Source: three-view drawing plus pictorial views. Frame: mm from the lowest corner of the part. A direction names the side the tool comes from. Round coordinates to 2 decimals unless told otherwise and drop trailing zeros. Loops run counter-clockwise (first coordinate to the right, second up) from the corner with the lowest first, then second, coordinate; pieces in that order, holes last. Notation, with made-up numbers: (29, 30) -> (66, 30) arc R27 ccw to (66, 49) -> close; hole circle Ø3 at (31.5, 58). An arc over 180 degrees is marked (long way). One line per question, with ' | ' between items. Start each with the question number.
Q1. Cut plane B-B on x = 17. Return loops of the section in (y, z).
Q2. Material intervals for L1, parallel to X at y = 2.25, z = 11.75; L2, parallel to Z at x = 21.75, y = 7.5; L3, parallel to Z at x = 9.5, y = 2.5, sorted ascending.
Q3. Access query for the marked faces 1, 2 and 3. Directions: +Z, -Z, +X, -X, +Y, -Y. A direction counts if a zero-diameter tool reaches every point of the face in a straight line with its end or side. Return the directions, or none.
Q4. Cut plane C-C on z = 4.75. Return loops of the section in (x, y).
Q5. Mould query, pull axis X, two halves, no side actions, for the marked faces 4, 5, 6 and 7. Classes: pulls with the +X half, pulls with the -X half, needs draft (parallel to the pull), parting line crosses it, or undercut.
Q6. Contact query for flat-ended pins moving along their axis: P1, Ø3.5, axis at y = 9.5, z = 7.5, coming from the -X side; P2, Ø1.5, axis at x = 2.5, z = 15.5, coming from the +Y side; P3, Ø1.5, axis at x = 11.5, z = 12, coming from the +Y side; P4, Ø6, axis at x = 15.5, y = 4.5, coming from the -Z side. Output: stop coordinate, or through.
Q7. Cut plane A-A on y = 5. Return loops of the section in (x, z), and give its area (3 significant figures).
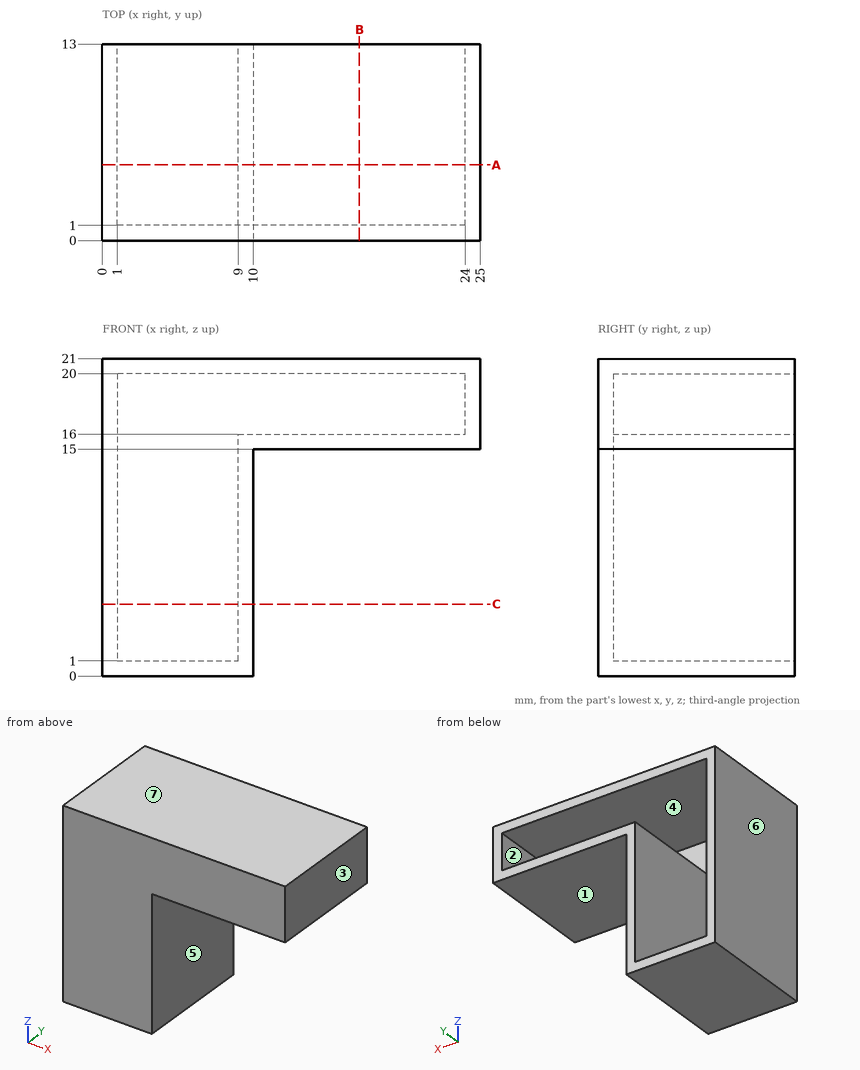
Results:
1) outline: (0, 15) -> (13, 15) -> (13, 16) -> (1, 16) -> (1, 20) -> (13, 20) -> (13, 21) -> (0, 21) -> close
2) L1: 0 to 1, 9 to 10 | L2: 15 to 16, 20 to 21 | L3: 0 to 16, 20 to 21
3) face 1: -Z, +X, +Y, -Y | face 2: +Y | face 3: +Z, -Z, +X, +Y, -Y
4) outline: (0, 0) -> (10, 0) -> (10, 13) -> (9, 13) -> (9, 1) -> (1, 1) -> (1, 13) -> (0, 13) -> close
5) face 4: undercut | face 5: pulls with the +X half | face 6: pulls with the -X half | face 7: needs draft
6) P1: x = 0 | P2: y = 1 | P3: through | P4: z = 15
7) outline: (0, 0) -> (10, 0) -> (10, 15) -> (25, 15) -> (25, 21) -> (0, 21) -> close; hole (1, 1) -> (9, 1) -> (9, 16) -> (24, 16) -> (24, 20) -> (1, 20) -> close | area: 88.0 mm^2
